```python
from build123d import *

# Parameters (mm, degrees)
SKETCH1_W           = 54
SKETCH1_H           = 54
BOSS_EXTRUDE1_DEPTH = 1.6
SKETCH2_R           = 1.5
CUT_EXTRUDE1_DEPTH  = 39.217273581
SKETCH3_W           = 4.2
SKETCH3_H           = 3.2
BOSS_EXTRUDE2_DEPTH = 1.2
SKETCH4_W           = 16
SKETCH4_H           = 7.6
BOSS_EXTRUDE3_DEPTH = 5.5
SKETCH5_W           = 10
SKETCH5_H           = 4
BOSS_EXTRUDE4_DEPTH = 3.2


with BuildPart() as part:
    # Sketch1 → Boss-Extrude1 (new body)
    with BuildSketch(Plane.YZ):
        Rectangle(SKETCH1_W, SKETCH1_H)
    extrude(amount=BOSS_EXTRUDE1_DEPTH)

    # Sketch2 → Cut-Extrude1 (cut, through all)
    with BuildSketch(Plane.YZ.offset(1.6)):
        with Locations(Location((-21.213203436, 21.213203436, 0), (0, 0, 270))):
            Circle(SKETCH2_R)
        with Locations(Location((21.213203436, 21.213203436, 0), (0, 0, 270))):
            Circle(SKETCH2_R)
        with Locations(Location((-21.213203436, -21.213203436, 0), (0, 0, 270))):
            Circle(SKETCH2_R)
        with Locations(Location((21.213203436, -21.213203436, 0), (0, 0, 270))):
            Circle(SKETCH2_R)
    extrude(amount=-CUT_EXTRUDE1_DEPTH, mode=Mode.SUBTRACT)

    # Sketch3 → Boss-Extrude2 (add)
    with BuildSketch(Plane(origin=(0, 0, 0), x_dir=(0, -1, 0), z_dir=(-1, 0, 0))):
        Rectangle(SKETCH3_W, SKETCH3_H)
    extrude(amount=BOSS_EXTRUDE2_DEPTH)

    # Sketch4 → Boss-Extrude3 (add)
    with BuildSketch(Plane.YZ.offset(1.6)):
        with Locations((0, -23.2)):
            Rectangle(SKETCH4_W, SKETCH4_H)
    extrude(amount=BOSS_EXTRUDE3_DEPTH)

    # Sketch5 → Boss-Extrude4 (add)
    with BuildSketch(Plane.YZ.offset(1.6)):
        with Locations((0, 25)):
            Rectangle(SKETCH5_W, SKETCH5_H)
    extrude(amount=BOSS_EXTRUDE4_DEPTH)


solid = part.part
```
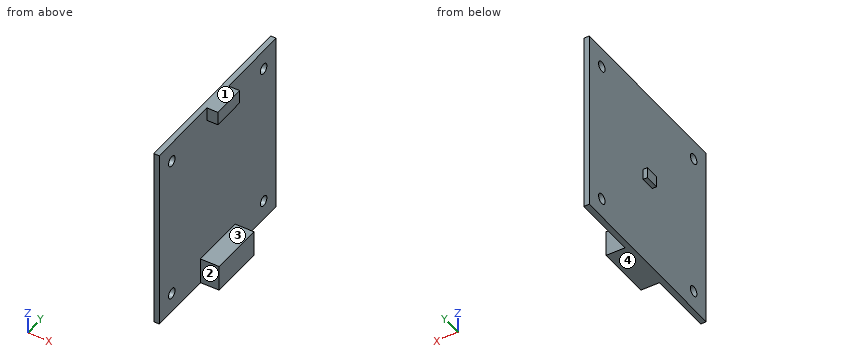
Source: CAD feature listing. Evaluate the final solid. Frame: model axes, mm. Face numbers are marked on the shaded views. Coordinates: 2 decimals unless noted, no trailing zeros. Loops run counter-clockwise (first coordinate to the right, second up) from the corner with the lowest first, then second, coordinate; pieces in that order, holes last. Notation, with made-up numbers: (-4, 42.25) -> (0, 42.25) arc R10 cw to (0, 52.25) -> close; hole circle Ø7 at (77.25, 82.5). An arc over 180 degrees is marked (long way). One line per item, written item: value. Start each with the question number.
Q1. Mould query, pull axis Z, two halves, no side actions, for the marked faces 1, 2, 3 and 4. Classes: pulls with the +Z half, pulls with the -Z half, needs draft (parallel to the pull), parting line crosses it, or undercut.
Q2. Line query: line 1 along Z through (x, y) = (4.25, 2); line 2 along Y through (x, z) = (0.5, -20); line 3 along X through (y, z) = (23, 17). Output: solid intervals per line, ascending.
Q3. Contact query for flat-ended pins moving along their axis: P1, Ø4, axis at y = -21.21, z = -21.21, coming from the -X side; P2, Ø2.5, axis at x = 4, z = 25, coming from the -Y side; P3, Ø1.6, axis at x = 4, z = -22.5, coming from the -Y side; P4, Ø1.6, axis at x = 5.5, y = 2, coming from the +Z side. Output: stop coordinate, or through.
Q4. Section query C-C, the plane y = -20.5. Return the cut outline in (x, z).
Q5. Section query B-B, the plane y = -4. Return the cut outline in (x, z), and give its area (3 significant figures).
Q6. Section query A-A, the plane x = 4. Return the cut outline in (y, z), and give its area (3 significant figures).
Q7. Section query D-D, the plane z = 24. Return the cut outline in (x, y).
Results:
1. face 1: pulls with the +Z half
1. face 2: needs draft
1. face 3: undercut
1. face 4: pulls with the -Z half
2. line 1: -27 to -19.4, 23 to 27
2. line 2: -27 to -22.1, -20.33 to 20.33, 22.1 to 27
2. line 3: 0 to 1.6
3. P1: x = 0
3. P2: y = -5
3. P3: y = -8
3. P4: z = 27
4. outline: (0, -27) -> (1.6, -27) -> (1.6, -22.53) -> (0, -22.53) -> close; (0, -19.89) -> (1.6, -19.89) -> (1.6, 19.89) -> (0, 19.89) -> close; (0, 22.53) -> (1.6, 22.53) -> (1.6, 27) -> (0, 27) -> close
5. outline: (0, -27) -> (7.1, -27) -> (7.1, -19.4) -> (1.6, -19.4) -> (1.6, 23) -> (4.8, 23) -> (4.8, 27) -> (0, 27) -> close
5. area: 141 mm^2
6. outline: (-8, -27) -> (8, -27) -> (8, -19.4) -> (-8, -19.4) -> close; (-5, 23) -> (5, 23) -> (5, 27) -> (-5, 27) -> close
6. area: 162 mm^2
7. outline: (0, -27) -> (1.6, -27) -> (1.6, -5) -> (4.8, -5) -> (4.8, 5) -> (1.6, 5) -> (1.6, 27) -> (0, 27) -> close
